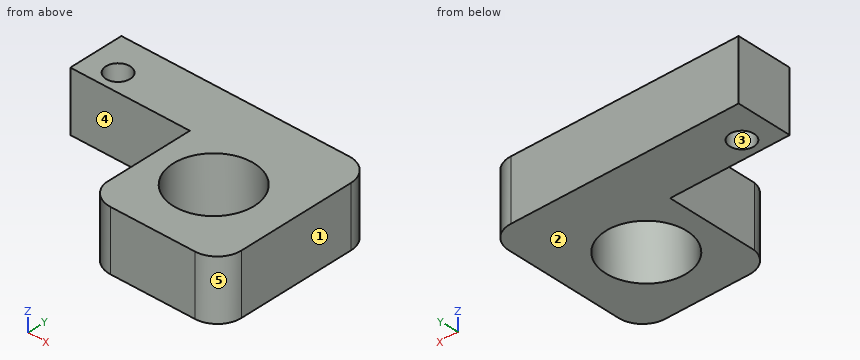
Autodesk Inventor part; units mm, degrees
ref_plane "YZ Plane" through (0, 0, 0) normal (1, 0, 0) x (0, 1, 0)
ref_plane "XZ Plane" through (0, 0, 0) normal (0, 1, 0) x (-1, 0, 0)
ref_plane "XY Plane" through (0, 0, 0) normal (0, 0, 1) x (1, 0, 0)
sketch "Skizze1" plane through (0, 0, 0) normal (0, 0, 1) x (1, 0, 0)
  circle A0 centre (2.5, -3) radius 0.5
  line L0 (0, 0) -> (0, -6)
  line L1 (0, -6) -> (5, -6)
  line L2 (5, 0) -> (5, -6)
  line L3 (0, 0) -> (5, 0)
  circle A1 centre (14.8779, -7.8108) radius 3.9802
  line L4 (5, 0) -> (18.8779, 0)
  line L5 (20.8779, -2) -> (20.8779, -11.8108)
  line L6 (18.8779, -13.8108) -> (11.8779, -13.8108)
  line L7 (9.8779, -11.8108) -> (9.8779, -6)
  line L8 (9.8779, -6) -> (5, -6)
  arc A2 (9.8779, -11.8108) -> (11.8779, -13.8108) centre (11.8779, -11.8108) ccw
  arc A3 (18.8779, -13.8108) -> (20.8779, -11.8108) centre (18.8779, -11.8108) ccw
  arc A4 (20.8779, -2) -> (18.8779, 0) centre (18.8779, -2) ccw
  line L9 (0, -4.579) -> (9.9072, -4.579)
  line L10 (9.9072, -4.579) -> (9.9072, -13.8108)
  line L11 (9.9072, -13.8108) -> (11.8779, -13.8108)
  circle A5 centre (2.5, -3) radius 1
  circle A6 centre (14.8779, -7.8108) radius 3.35
  point P0 (9.9072, -12.1516)
  dimension "d0" = 6
  dimension "d1" = 5
  dimension "d2" = 6
  dimension "d3" = 2
  dimension "d9" = 2
  dimension "d10" = 6.7
extrude "Extrusion1" add sketch "Skizze1" along normal blind 5 contours L3 L2 L9 L0 | L4 A4 L5 A3 L6 A2 L10 L9 L2 | A1
properties part number "IM_Lensholder_motorized_lensadapter"
CAD build for the part. Positions are in the model's coordinates, mm. Face numbers are marked on the shaded views. A direction names the side the tool comes from. Round coordinates to 2 decimals unless told otherwise and drop trailing zeros. Order: outer loops, then holes, each group sorted by start corner. A loop starts at its lowest first (then second) coordinate and runs counter-clockwise, first axis right, second up.
Q1. Wall check: L1, parallel to Y at x = 2.5, z = 1.6; L2, parallel to X at y = -6.25, z = 3.7; L3, parallel to X at y = -7.25, z = 3.55. Give the ranges that are in metal, low to high.
Q2. Slice it at C-C (z = 1). Write the cut outline in (x, y).
Q3. Which spindle directions (+Z, -Z, +X, -X, +Y, -Y) get a long thin tool onto all of the face, cutting with end or side? Do the marked faces 4 and 5. Say none if no direction does.
Q4. Two-plate mould, pull along X, no slides. Class the marked faces 1, 2 and 3: pulls with the +X half, pulls with the -X half, needs draft (parallel to the pull), parting line crosses it, or undercut.
Q5. Drop flat-ended pins along their axis: pin 1 (1.8 mm diameter, centred on x = 2.5, y = -3, fed in from +Z); pin 2 (1.5 mm diameter, centred on x = 6, z = 1.5, fed in from -Y). Give the stop position or say it passes through.
Q6. Slice it at A-A (y = -3). Write the cut outline in (x, z), and give its area (3 significant figures).
Q7. Slice it at B-B (x = 2.5). Write the cut outline in (y, z), and give its area (3 significant figures).
Q8. Slice it at D-D (x = 8.75). Write the cut outline in (y, z), and give its area (3 significant figures).
Results below:
1. L1: y = -4.58 to -4, -2 to 0
1. L2: x = 9.91 to 11.91, 17.84 to 20.88
1. L3: x = 9.91 to 11.58, 18.18 to 20.88
2. outline: (0, -4.58) - (9.91, -4.58) - (9.91, -12.15) arc R2 ccw to (11.88, -13.81) - (18.88, -13.81) arc R2 ccw to (20.88, -11.81) - (20.88, -2) arc R2 ccw to (18.88, 0) - (0, 0) - close; hole circle Ø2 at (2.5, -3); hole circle Ø6.7 at (14.88, -7.81)
3. face 4: +Z, -Z, -X, -Y
3. face 5: +Z, -Z, +X, -Y
4. face 1: pulls with the +X half
4. face 2: needs draft
4. face 3: undercut
5. pin 1: passes through
5. pin 2: stops at y = -4.58
6. outline: (0, 0) - (1.5, 0) - (1.5, 5) - (0, 5) - close; (3.5, 0) - (20.88, 0) - (20.88, 5) - (3.5, 5) - close
6. area: 94.4 mm2
7. outline: (-4.58, 0) - (-4, 0) - (-4, 5) - (-4.58, 5) - close; (-2, 0) - (0, 0) - (0, 5) - (-2, 5) - close
7. area: 12.9 mm2
8. outline: (-4.58, 0) - (0, 0) - (0, 5) - (-4.58, 5) - close
8. area: 22.9 mm2
